```python
from build123d import *

# Parameters (mm, degrees)
SKETCH2_W           = 100
SKETCH2_H           = 55
BOSS_EXTRUDE1_DEPTH = 15
CUT_EXTRUDE2_DEPTH  = 76.828754441
SKETCH9_R           = 16.637
CUT_EXTRUDE3_DEPTH  = 70.869600016
CUT_EXTRUDE4_DEPTH  = 76.828754441
CUT_EXTRUDE5_DEPTH  = 76.828754441
SKETCH12_W          = 91
SKETCH12_H          = 35
CUT_EXTRUDE6_DEPTH  = 7


with BuildPart() as part:
    # Sketch2 → Boss-Extrude1 (new, symmetric)
    with BuildSketch(Plane.XY):
        Rectangle(SKETCH2_W, SKETCH2_H)
    extrude(amount=BOSS_EXTRUDE1_DEPTH, both=True)

    # Sketch5 → Cut-Extrude2 (cut, through all)
    with BuildSketch(Plane(origin=(0, 27.5, 0), x_dir=(1, 0, 0), z_dir=(0, 1, 0))):
        with BuildLine():
            ThreePointArc((-38.188858584, 4.386875892), (-38.44, 0), (-38.188858584, -4.386875892))
            ThreePointArc((-38.188858584, -4.386875892), (-34.434130699, -7.367851993), (-31.453154598, -3.613124108))
            ThreePointArc((-31.453154598, -3.613124108), (-31.66, 0), (-31.453154598, 3.613124108))
            ThreePointArc((-31.453154598, 3.613124108), (-34.434130699, 7.367851993), (-38.188858584, 4.386875892))
        make_face()
        with BuildLine():
            ThreePointArc((38.188858584, -4.386875892), (38.44, 0), (38.188858584, 4.386875892))
            ThreePointArc((38.188858584, 4.386875892), (34.434130699, 7.367851993), (31.453154598, 3.613124108))
            ThreePointArc((31.453154598, 3.613124108), (31.66, 0), (31.453154598, -3.613124108))
            ThreePointArc((31.453154598, -3.613124108), (34.434130699, -7.367851993), (38.188858584, -4.386875892))
        make_face()
    extrude(amount=-CUT_EXTRUDE2_DEPTH, mode=Mode.SUBTRACT)

    # Sketch9 → Cut-Extrude3 (cut, through all)
    with BuildSketch(Plane(origin=(0, 5.592150698, -20.870190528), x_dir=(-1, 0, 0), z_dir=(0, 0.25881904510252135, -0.9659258262890681))):
        with Locations(Location((0, 2, 0), (0, 0, 90))):
            Circle(SKETCH9_R)
    extrude(amount=-CUT_EXTRUDE3_DEPTH, mode=Mode.SUBTRACT)

    # Sketch10 → Cut-Extrude4 (cut, through all)
    with BuildSketch(Plane(origin=(0, 27.5, 0), x_dir=(1, 0, 0), z_dir=(0, 1, 0))):
        Polygon((50, 5), (50, 15), (38, 15), align=None)
        Polygon((50, -15), (50, -5), (38, -15), align=None)
        Polygon((-38, -15), (-50, -5), (-50, -15), align=None)
        Polygon((-50, 5), (-38, 15), (-50, 15), align=None)
    extrude(amount=-CUT_EXTRUDE4_DEPTH, mode=Mode.SUBTRACT)

    # Sketch11 → Cut-Extrude5 (cut, through all)
    with BuildSketch(Plane(origin=(0, 27.5, 0), x_dir=(1, 0, 0), z_dir=(0, 1, 0))):
        Polygon((-42.5, 11.25), (-42.5, -11.25), (-50, -5), (-50, 5), align=None)
        Polygon((42.5, 11.25), (42.5, -11.25), (50, -5), (50, 5), align=None)
    extrude(amount=-CUT_EXTRUDE5_DEPTH, mode=Mode.SUBTRACT)

    # Sketch12 → Cut-Extrude6 (cut)
    with BuildSketch(Plane.XZ.offset(27.5)):
        Rectangle(SKETCH12_W, SKETCH12_H)
    extrude(amount=-CUT_EXTRUDE6_DEPTH, mode=Mode.SUBTRACT)


solid = part.part
```
The listing builds one solid part. Answer for the finished solid, in the listing's coordinates (mm). A direction names the side the tool comes from. Give positions to 0.01 mm unless a question says otherwise; leave off trailing zeros. Return JSON: item names as keys, results as strings. Group by question number.
1. Determine the mould class of faces 3 (the flat face through (-1, -20.5, 0)), 4 (the cylindrical face through (-38.44, 3.84, -0.06)), 5 (the flat face through (40.22, 3.84, -13.15)) for opening direction X: pulls with the +X half, pulls with the -X half, needs draft (parallel to the pull), parting line crosses it, or undercut.
2. Straight lines are drawn through the part: line 1 (X direction, y = 5, z = -4.5); line 2 (X direction, y = -4, z = 1); line 3 (X direction, y = 18.5, z = -8). For each, find the intervals that lie inside material, in ascending order. Write a range as [from, to].
3. Which of the six approach directions +Z, -Z, +X, -X, +Y, -Y give full straight-line access (tool end or side, diameter ignored) to faces 1 (the cylindrical face through (-34.36, 3.84, -7.36)), 2 (the flat face through (-40.22, 3.84, 13.15))?
4. Find section A-A (z = 6.5). State how many separate pieces and enclosed holes the cut face has, then the cut area to 3 significant figures.
Verdict:
{
 "1": {"face 3": "needs draft", "face 4": "undercut", "face 5": "pulls with the +X half"},
 "2": {"line 1": "x = [-42.5, -38.17], [-31.47, -16.55], [16.55, 31.47], [38.17, 42.5]", "line 2": "x = [-42.5, -38.43], [-31.64, -15.66], [15.66, 31.64], [38.43, 42.5]", "line 3": "x = [-42.5, -9.29], [9.29, 42.5]"},
 "3": {"face 1": "+Y, -Y", "face 2": "+Z, -X, +Y, -Y"},
 "4": {"separate pieces": "3", "enclosed holes": "1", "area": "2,740 mm^2"}
}
